Work out the finished part from the listing and answer in its coordinate system (mm). A direction names the side the tool comes from. Coordinates: 2 decimals unless noted, no trailing zeros. Order: outer loops, then holes, each group sorted by start corner. A loop starts at its lowest first (then second) coordinate and runs counter-clockwise, first axis right, second up. Notation, with made-up numbers: (45, 36.5) - (70, 36.5) arc R14 ccw to (70, 48.5) - close; hole circle Ø1 at (80, 65). An arc over 180 degrees is marked (long way). Answer as a JSON object with one key per item and string values. Group by question number.
1) Find the intervals of material crossed by line 1 along Z through (x, y) = (-183, 101); line 2 along Z through (x, y) = (57.5, 160); line 3 along Y through (x, z) = (183, 12), in increasing order.
2) The mould has two halves that part along Y. Classify faces 5 (the face through (-12.7, -842, 88)), 6 (the face through (0, -1016, 189)), 7 (the face through (-12.7, -460, 13)): released by +Y, released by -Y, zero draft, split by the parting line, or undercut.
3) Section C-C (y = 178) is taken. Give the vertices of the cut face in (x, z), plus the area to 3 significant figures.
4) Section B-B (y = -771) is taken. Give the vertices of the cut face in (x, z) (3 decimals), plus the area to 3 significant figures.
5) Each of these flat-tipped pins is pushed along its axis until it touches: P1, Ø12.5, axis at y = -458, z = 9, coming from the -X side; P2, Ø7.5, axis at x = -97, z = 13, coming from the -Y side; P3, Ø9.5, axis at x = 1.5, z = 180.5, coming from the -Y side. Where does it stop, or does it pass through?
6) Section A-A (z = 101) is taken. Give the vertices of the cut face in (x, y) (3 decimals).
7) Section D-D (z = 336.5) is taken. Give the vertices of the cut face in (x, y) (3 decimals).
8) A tool of negligible diameter and unlimited length cuts with its end or side. For faces 1 (the face through (0, -355.6, 226)), 2 (the face through (0, -331, 431.8)), 3 (the face through (-12.7, -343, 226)), 4 (the face through (126, -12.7, 13)), from which of +Z, -Z, +X, -X, +Y, -Y can it reach the whole face along a straight path? Write none if from no direction.
from build123d import *

# Parameters (mm, degrees)
F0_W      = 406.4
F0_H      = 711.2
F0_W_2    = 101.6
F0_H_2    = 317.5
F0_H_3    = 660.4
F1_DEPTH  = 25.4
F2_W      = 25.4
F2_H      = 25.4
F2_W_2    = 19.05
F2_H_2    = 19.05
F3_DEPTH  = 406.4
F4_R      = 7.9375
F5_DEPTH  = 25.4
F6_R      = 7.9375
F7_DEPTH  = 25.4
F8_W      = 25.4
F8_H      = 25.4
F8_W_2    = 19.05
F8_H_2    = 19.05
F9_DEPTH  = 508
F10_W     = 25.4
F10_H     = 25.4
F10_W_2   = 19.05
F10_H_2   = 19.05
F11_DEPTH = 165.1
F12_W     = 25.4
F12_H     = 25.4
F12_W_2   = 19.05
F12_H_2   = 19.05
F13_DEPTH = 152.4
F15_DEPTH = 25.4


with BuildPart() as f1:
    # F0 (on Top) → F1 (new body)
    with BuildSketch(Plane.XY):
        Rectangle(F0_W, F0_H)
        with Locations((-127, -171.45)):
            Rectangle(F0_W_2, F0_H_2, mode=Mode.SUBTRACT)
        with Locations((127, -171.45)):
            Rectangle(F0_W_2, F0_H_2, mode=Mode.SUBTRACT)
        with Locations((-127, 171.45)):
            Rectangle(F0_W_2, F0_H_2, mode=Mode.SUBTRACT)
        Rectangle(F0_W_2, F0_H_3, mode=Mode.SUBTRACT)
        with Locations((127, 171.45)):
            Rectangle(F0_W_2, F0_H_2, mode=Mode.SUBTRACT)
    extrude(amount=F1_DEPTH)

    # F2 (on face) → F3 (join)
    with BuildSketch(Plane.XY.offset(25.4)):
        with Locations((0, -342.9)):
            Rectangle(F2_W, F2_H)
        with Locations((0, -342.9)):
            Rectangle(F2_W_2, F2_H_2, mode=Mode.SUBTRACT)
    extrude(amount=F3_DEPTH)

    # F4 (on face) → F5 (cut)
    with BuildSketch(Plane.YZ.offset(203.2)):
        with Locations((101.6, 12.7)):
            Circle(F4_R)
    extrude(amount=-F5_DEPTH, mode=Mode.SUBTRACT)

    # F6 (on face) → F7 (cut)
    with BuildSketch(Plane(origin=(-203.2, 0, 0), x_dir=(0, -1, 0), z_dir=(-1, 0, 0))):
        with Locations((-101.6, 12.7)):
            Circle(F6_R)
    extrude(amount=-F7_DEPTH, mode=Mode.SUBTRACT)

    # F8 (on face) → F9 (join)
    with BuildSketch(Plane.XZ.offset(355.6)):
        with Locations((0, 12.7)):
            Rectangle(F8_W, F8_H)
        with Locations((0, 12.7)):
            Rectangle(F8_W_2, F8_H_2, mode=Mode.SUBTRACT)
    extrude(amount=F9_DEPTH)

    # F10 (on face) → F11 (join)
    with BuildSketch(Plane.XY.offset(25.4)):
        with Locations((0, -850.9)):
            Rectangle(F10_W, F10_H)
        with Locations((0, -850.9)):
            Rectangle(F10_W_2, F10_H_2, mode=Mode.SUBTRACT)
    extrude(amount=F11_DEPTH)

    # F12 (on face) → F13 (join)
    with BuildSketch(Plane.XZ.offset(863.6)):
        with Locations((0, 177.8)):
            Rectangle(F12_W, F12_H)
        with Locations((0, 177.8)):
            Rectangle(F12_W_2, F12_H_2, mode=Mode.SUBTRACT)
    extrude(amount=F13_DEPTH)

    # F14 (on Top) → F15 (join)
    with BuildSketch(Plane.XY):
        Polygon((-171.45, -355.6), (-203.2, -355.6), (-12.7, -609.6), (-12.7, -567.266667), align=None)
        Polygon((12.7, -609.6), (203.2, -355.6), (171.45, -355.6), (12.7, -567.266667), align=None)
    extrude(amount=F15_DEPTH)


solid = f1.part
Report:
{
 "1": {"line 1": "z = 0 to 4.79, 20.61 to 25.4", "line 2": "z = 0 to 25.4", "line 3": "y = -382.53 to 93.69, 109.51 to 355.6"},
 "2": {"face 5": "zero draft", "face 6": "released by -Y", "face 7": "undercut"},
 "3": {"outline": "(-203.2, 0) - (-177.8, 0) - (-177.8, 25.4) - (-203.2, 25.4) - close; (-76.2, 0) - (-50.8, 0) - (-50.8, 25.4) - (-76.2, 25.4) - close; (50.8, 0) - (76.2, 0) - (76.2, 25.4) - (50.8, 25.4) - close; (177.8, 0) - (203.2, 0) - (203.2, 25.4) - (177.8, 25.4) - close", "area": "2,580 mm²"},
 "4": {"outline": "(-12.7, 0) - (12.7, 0) - (12.7, 25.4) - (-12.7, 25.4) - close; hole (-9.525, 3.175) - (9.525, 3.175) - (9.525, 22.225) - (-9.525, 22.225) - close", "area": "282 mm²"},
 "5": {"P1": "stops at x = -131.09", "P2": "stops at y = -502.2", "P3": "stops at y = -863.6"},
 "6": {"outline": "(-12.7, -863.6) - (12.7, -863.6) - (12.7, -838.2) - (-12.7, -838.2) - close; (-12.7, -355.6) - (12.7, -355.6) - (12.7, -330.2) - (-12.7, -330.2) - close; hole (-9.525, -860.425) - (9.525, -860.425) - (9.525, -841.375) - (-9.525, -841.375) - close; hole (-9.525, -352.425) - (9.525, -352.425) - (9.525, -333.375) - (-9.525, -333.375) - close"},
 "7": {"outline": "(-12.7, -355.6) - (12.7, -355.6) - (12.7, -330.2) - (-12.7, -330.2) - close; hole (-9.525, -352.425) - (9.525, -352.425) - (9.525, -333.375) - (-9.525, -333.375) - close"},
 "8": {"face 1": "+Z, +X, -X", "face 2": "+Z, +X, -X, +Y, -Y", "face 3": "+Z, -X, +Y, -Y", "face 4": "+Z, -Z"}
}
